Part print with two shaded views. Sizes in mm from the minimum x, y, z corner. Round coordinates to 2 decimals unless told otherwise and drop trailing zeros. Write each loop counter-clockwise with the first axis right and the second up, starting at its lowest first coordinate (ties: lowest second). Pieces come first, ordered by that corner, then holes.
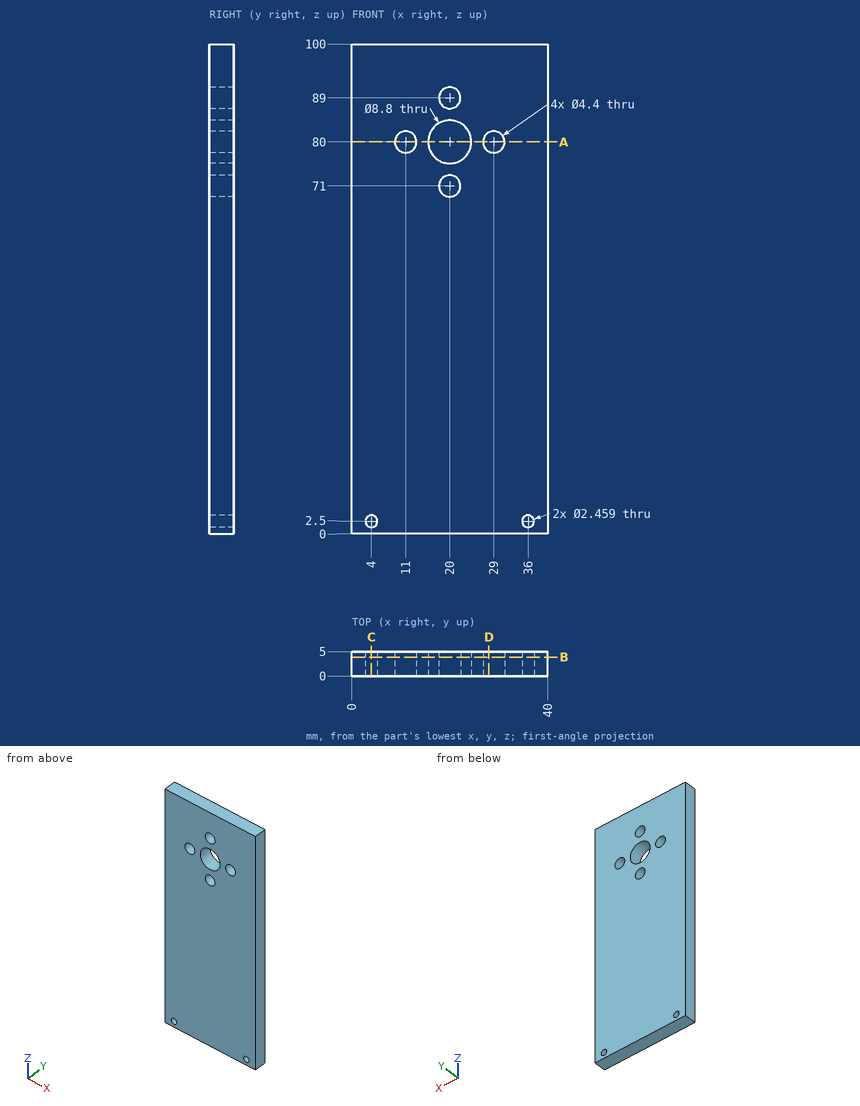
Q1. Cut at D-D on x = 28. Write the cut outline in (y, z).
Values follow:
outline: (0, 0) - (5, 0) - (5, 78.04) - (0, 78.04) - close; (0, 81.96) - (5, 81.96) - (5, 100) - (0, 100) - close
Q2. Cut at C-C on x = 4. Write the cut outline in (y, z).
Values follow:
outline: (0, 0) - (5, 0) - (5, 1.27) - (0, 1.27) - close; (0, 3.73) - (5, 3.73) - (5, 100) - (0, 100) - close
Q3. Cut at A-A on z = 80. Write the cut outline in (x, y).
Values follow:
outline: (0, 0) - (8.8, 0) - (8.8, 5) - (0, 5) - close; (13.2, 0) - (15.6, 0) - (15.6, 5) - (13.2, 5) - close; (24.4, 0) - (26.8, 0) - (26.8, 5) - (24.4, 5) - close; (31.2, 0) - (40, 0) - (40, 5) - (31.2, 5) - close
Q4. Cut at B-B on y = 3.85. Write the cut outline in (x, z).
Values follow:
outline: (0, 0) - (40, 0) - (40, 100) - (0, 100) - close; hole circle Ø2.46 at (4, 2.5); hole circle Ø4.4 at (11, 80); hole circle Ø8.8 at (20, 80); hole circle Ø4.4 at (20, 71); hole circle Ø4.4 at (20, 89); hole circle Ø4.4 at (29, 80); hole circle Ø2.46 at (36, 2.5)
Q5. Wall check: L1, parallel to X at y = 3.8, z = 80; L2, parallel to Z at x = 20, y = 2.95; L3, parallel to X at y = 3.6, z = 89. Give the ranges that are in metal, low to high.
Values follow:
L1: x = 0 to 8.8, 13.2 to 15.6, 24.4 to 26.8, 31.2 to 40
L2: z = 0 to 68.8, 73.2 to 75.6, 84.4 to 86.8, 91.2 to 100
L3: x = 0 to 17.8, 22.2 to 40
